The listing builds one solid part. Answer for the finished solid, in the listing's coordinates (mm). A direction names the side the tool comes from. Give positions to 0.01 mm unless a question says otherwise; leave off trailing zeros. Write each loop counter-clockwise with the first axis right and the second up, starting at its lowest first coordinate (ties: lowest second). Pieces come first, ordered by that corner, then holes. Notation, with made-up numbers: (47, 36) - (84, 36) arc R21 cw to (84, 58) - close; hole circle Ø5 at (-28.5, 41.25). An arc over 180 degrees is marked (long way). Return JSON: item names as keys, results as strings.
Autodesk Fusion 360 part; units mm, degrees
sketch "Boceto1" plane through (0, 0, 0) normal (0, 0, 1) x (1, 0, 0)
  circle A0 centre (0, 9) radius 13
  circle A1 centre (0, -9) radius 13
  line L0 (-13, -9) -> (-13, 9)
  line L1 (13, -9) -> (13, 9)
extrude "Extruir1" add sketch "Boceto1" along normal blind 8 makes body 1
sketch "Boceto2" plane through (0, 0, 0) normal (0, 0, 1) x (1, 0, 0)
  circle A0 centre (0, 9) radius 8.6
  circle A1 centre (0, -9) radius 8.6
  line L0 (-8.6, -9) -> (-8.6, 9)
  line L1 (8.6, -9) -> (8.6, 9)
extrude "Extruir2" cut sketch "Boceto2" along normal blind 1.5 bodies 1
sketch "Boceto3" plane through (0, 0, 0) normal (0, 0, 1) x (1, 0, 0)
  circle A0 centre (0, 9) radius 8.2
  circle A1 centre (0, -9) radius 8.2
extrude "Extruir3" cut sketch "Boceto3" along normal blind 3.7 bodies 1
sketch "Boceto4" plane through (0, 0, 0) normal (0, 0, 1) x (1, 0, 0)
  line L0 (-6.5, -15.5) -> (6.5, -15.5)
  line L1 (6.5, -15.5) -> (6.5, -2.5)
  line L2 (6.5, -2.5) -> (-6.5, -2.5)
  line L3 (-6.5, -2.5) -> (-6.5, -15.5)
extrude "Extruir4" cut sketch "Boceto4" along normal blind 8 bodies 1
sketch "Boceto5" plane through (0, 0, 0) normal (0, 0, 1) x (1, 0, 0)
  circle A0 centre (0, 9) radius 13
  circle A1 centre (0, -9) radius 13
  line L0 (-13, -9) -> (-13, 9)
  line L1 (13, -9) -> (13, 9)
extrude "Extruir5" add sketch "Boceto5" along normal blind 8 separate body makes body 2
sketch "Boceto6" plane through (0, 0, 0) normal (0, 0, 1) x (1, 0, 0)
  circle A0 centre (0, 9) radius 8.2
  circle A1 centre (0, -9) radius 8.2
  line L0 (-8.2, -9) -> (-8.2, 9)
  line L1 (8.2, -9) -> (8.2, 9)
extrude "Extruir6" cut sketch "Boceto6" along normal blind 1.5 bodies 2
sketch "Boceto7" plane through (0, 0, 0) normal (0, 0, 1) x (1, 0, 0)
  circle A0 centre (0, 9) radius 7.5
  circle A1 centre (0, -9) radius 7.5
extrude "Extruir7" cut sketch "Boceto7" along normal blind 3.7 bodies 2
sketch "Boceto8" plane through (0, 0, 0) normal (0, 0, 1) x (1, 0, 0)
  line L0 (-7, -16) -> (7, -16)
  line L1 (7, -16) -> (7, -2)
  line L2 (7, -2) -> (-7, -2)
  line L3 (-7, -2) -> (-7, -16)
extrude "Extruir8" cut sketch "Boceto8" along normal blind 8 bodies 2
sketch "Boceto9" plane through (0, 0, 0) normal (0, 0, 1) x (1, 0, 0)
  circle A0 centre (0, 9) radius 13
  circle A1 centre (0, -9) radius 13
  line L0 (-13, -9) -> (-13, 9)
  line L1 (13, -9) -> (13, 9)
extrude "Extruir9" add sketch "Boceto9" along normal blind 8 separate body makes body 3
sketch "Boceto10" plane through (0, 0, 0) normal (0, 0, 1) x (1, 0, 0)
  circle A0 centre (0, 9) radius 8.1
  circle A1 centre (0, -9) radius 8.1
  line L0 (-8.1, -9) -> (-8.1, 9)
  line L1 (8.1, -9) -> (8.1, 9)
extrude "Extruir10" cut sketch "Boceto10" along normal blind 1.5 bodies 3
sketch "Boceto11" plane through (0, 0, 0) normal (0, 0, 1) x (1, 0, 0)
  circle A0 centre (0, 9) radius 7.4
  circle A1 centre (0, -9) radius 7.4
extrude "Extruir11" cut sketch "Boceto11" along normal blind 3.7 bodies 3
sketch "Boceto12" plane through (0, 0, 0) normal (0, 0, 1) x (1, 0, 0)
  line L0 (-7, -16) -> (7, -16)
  line L1 (7, -16) -> (7, -2)
  line L2 (7, -2) -> (-7, -2)
  line L3 (-7, -2) -> (-7, -16)
extrude "Extruir12" cut sketch "Boceto12" along normal blind 8 bodies 3
hidden bodies 1 2
Item 1: A cutting plane is placed at C-C on y = 1. Determine the outline of the cut face in (x, z).
Answer below:
{"outline": "(-13, 0) - (-8.1, 0) - (-8.1, 1.5) - (8.1, 1.5) - (8.1, 0) - (13, 0) - (13, 8) - (-13, 8) - close"}
Item 2: A cutting plane is placed at D-D on z = 5. Determine the outline of the cut face in (x, y).
Answer below:
{"outline": "(-13, -9) arc R13 ccw to (13, -9) - (13, 9) arc R13 ccw to (-13, 9) - close; hole (-7, -16) - (7, -16) - (7, -2) - (-7, -2) - close"}
Item 3: A cutting plane is placed at B-B on z = 2. Determine the outline of the cut face in (x, y), then the cut area to 3 significant figures.
Answer below:
{"outline": "(-13, -9) arc R13 ccw to (13, -9) - (13, 9) arc R13 ccw to (-13, 9) - close; hole circle Ø14.8 at (0, 9); hole (-7, -16) - (-2.4, -16) arc R7.4 ccw to (2.4, -16) - (7, -16) - (7, -11.4) arc R7.4 ccw to (7, -6.6) - (7, -2) - (2.4, -2) arc R7.4 ccw to (-2.4, -2) - (-7, -2) - (-7, -6.6) arc R7.4 ccw to (-7, -11.4) - close", "area": "626 mm²"}
Item 4: Flat-ended cylindrical pins translate along their axes: P1, Ø3, axis at x = 2.5, y = -13.5, coming from the +Z side; P2, Ø2, axis at x = 1, z = 3, coming from the -Y side; P3, Ø3, axis at x = -9, z = 4, coming from the -Y side; P4, Ø4.5, axis at x = -1.5, y = 7.5, coming from the -Z side. Find the tip coordinate at first contact, or state that the pin passes through.
Answer below:
{"P1": "passes through", "P2": "stops at y = -22", "P3": "stops at y = -19.62", "P4": "stops at z = 3.7"}
Item 5: Consider L1, parallel to Y at x = 0, z = 2.05; L2, parallel to X at y = 9, z = 2.95; L3, parallel to X at y = 0.5, z = 1. Determine where each line is inside the solid, lowest interval first.
Answer below:
{"L1": "y = -22 to -16.4, -1.6 to 1.6, 16.4 to 22", "L2": "x = -13 to -7.4, 7.4 to 13", "L3": "x = -13 to -8.1, 8.1 to 13"}
Item 6: The mould has two halves that part along X. Classify faces 4 (the face through (-0.18, 17.1, 0.74)), 5 (the face through (-7.4, -9, 2.6)), 6 (the face through (0, 22, 4)), 7 (the face through (13, 0, 4)): +X half, -X half, draft (parallel to the pull), parting line (faces both ways), or undercut.
Answer below:
{"face 4": "undercut", "face 5": "undercut", "face 6": "parting line", "face 7": "+X half"}
Item 7: For faces 1 (the face through (-7.812, -11.14, 0.74)), 2 (the face through (8.5, 0.3, 0)), 3 (the face through (-7, -9, 5)), determine the directions among +Z, -Z, +X, -X, +Y, -Y from which every point of the face is accessible in a straight line to the end or side of a thin tool.
Answer below:
{"face 1": "-Z", "face 2": "-Z, +X, -X, +Y, -Y", "face 3": "+Z, -Z"}
Item 8: A cutting plane is placed at A-A on x = 0. Determine the outline of the cut face in (y, z), then the cut area to 3 significant figures.
Answer below:
{"outline": "(-22, 0) - (-17.1, 0) - (-17.1, 1.5) - (-16.4, 1.5) - (-16.4, 3.7) - (-16, 3.7) - (-16, 8) - (-22, 8) - close; (-2, 3.7) - (-1.6, 3.7) - (-1.6, 1.5) - (1.6, 1.5) - (1.6, 3.7) - (16.4, 3.7) - (16.4, 1.5) - (17.1, 1.5) - (17.1, 0) - (22, 0) - (22, 8) - (-2, 8) - close", "area": "175 mm²"}
